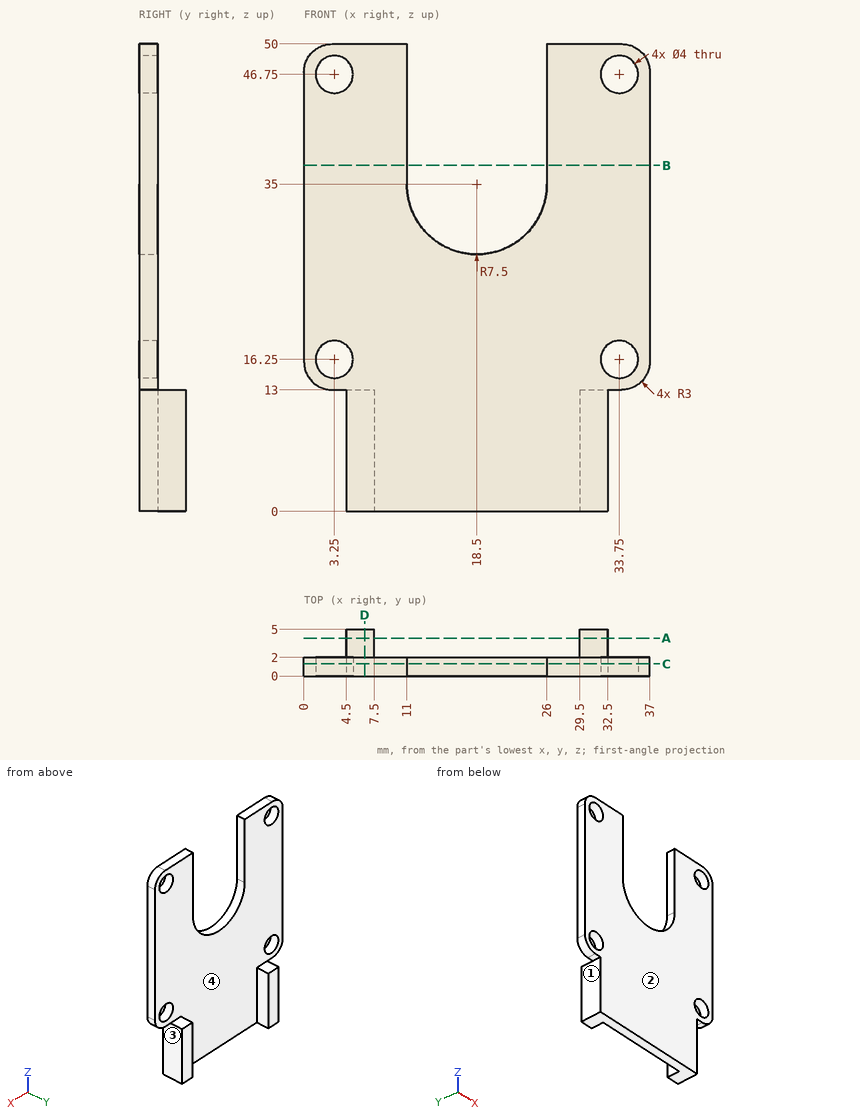
Can you work these out from the drawing? Everything is in mm from the part's minimum corner. Coordinates: 2 decimals unless noted, no trailing zeros. Order: outer loops, then holes, each group sorted by start corner. A loop starts at its lowest first (then second) coordinate and runs counter-clockwise, first axis right, second up. Notation, with made-up numbers: M 87,-25.5 L 128,-25.5 A5 ccw 128,-17.5 Z; hole C 77,51 d3. An arc over 180 degrees is marked long. Answer as CSV lines item,"result". Start each with the question number.
1. I want a section at C-C, the plane y = 1.3. Write out the boundary of the cut face in (x, z), and give its area (3 significant figures).
2. For pin 1 (0.8 mm diameter, centred on x = 4, y = 0.5, fed in from -Z); pin 2 (2.5 mm diameter, centred on x = 3.25, z = 46.75, fed in from -Y); pin 3 (1.5 mm diameter, centred on y = 3.5, z = 5, fed in from +X); pin 4 (4.5 mm diameter, centred on x = 3.25, z = 16.25, fed in from +Y), each with a flat end and sliding along its axis, tell me the tip position at first contact or that it passes through.
3. I want a section at A-A, the plane y = 4.05. Write out the boundary of the cut face in (x, z), and give its area (3 significant figures).
4. I need wall thicknesses on line 1 (X direction, y = 0.9, z = 16.25); line 2 (Z direction, x = 3.25, y = 0.95); line 3 (X direction, y = 1.1, z = 46.75). Which ranges of each line are inside material? Lowest first, please. Write a range as [from, to].
5. I want a section at B-B, the plane z = 37. Write out the boundary of the cut face in (x, y).
6. We'd pull the mould along X, two halves only. Please class the marked faces 1, 2, 3 and 4: released by +X, released by -X, zero draft, split by the parting line, or undercut.
7. I want a section at D-D, the plane x = 6.5. Write out the boundary of the cut face in (y, z).
Recorded:
1,outline,"M 0,16 A3 ccw 3,13 L 4.5,13 L 4.5,0 L 32.5,0 L 32.5,13 L 34,13 A3 ccw 37,16 L 37,47 A3 ccw 34,50 L 26,50 L 26,35 A7.5 cw 11,35 L 11,50 L 3,50 A3 ccw 0,47 Z; hole C 3.25,16.25 d4; hole C 3.25,46.75 d4; hole C 33.75,16.25 d4; hole C 33.75,46.75 d4"
1,area,"1,360 mm2"
2,pin 1,"stops at z = 13"
2,pin 2,"passes through"
2,pin 3,"stops at x = 32.5"
2,pin 4,"stops at y = 2"
3,outline,"M 4.5,0 L 7.5,0 L 7.5,13 L 4.5,13 Z; M 29.5,0 L 32.5,0 L 32.5,13 L 29.5,13 Z"
3,area,"78.0 mm2"
4,line 1,"x = [0, 1.25], [5.25, 31.75], [35.75, 37]"
4,line 2,"z = [13, 14.25], [18.25, 44.75], [48.75, 50]"
4,line 3,"x = [0, 1.25], [5.25, 11], [26, 31.75], [35.75, 37]"
5,outline,"M 0,0 L 11,0 L 11,2 L 0,2 Z; M 26,0 L 37,0 L 37,2 L 26,2 Z"
6,face 1,"released by -X"
6,face 2,"zero draft"
6,face 3,"released by +X"
6,face 4,"undercut"
7,outline,"M 0,0 L 5,0 L 5,13 L 2,13 L 2,50 L 0,50 Z"
